Autodesk Fusion 360 part; units mm, degrees
sketch "草图1" plane through (0, 0, 0) normal (1, 0, 0) x (0, 1, 0)
  circle A0 centre (0, 0) radius 5
  circle A1 centre (0, 0) radius 11
  line L0 (0, 11) -> (62.4602, 11)
  line L1 (62.4602, 11) -> (44, -11)
  line L2 (44, -11) -> (0, -11)
  line L3 (62.4602, 11) -> (67.0565, 7.1433)
  line L4 (67.0565, 7.1433) -> (48.5963, -14.8567)
  line L5 (48.5963, -14.8567) -> (44, -11)
  dimension "d1" = 22
  dimension "d2" = 10
  dimension "d3" = 44
  dimension "d4" = 130
  dimension "d5" = 6
extrude "拉伸1" add sketch "草图1" along normal blind 19 contours A1 makes body 1
extrude "拉伸2" add sketch "草图1" along normal blind 5 contours A1 L0 L1 L2 bodies 1
extrude "拉伸3" add sketch "草图1" along normal blind 18 contours L1 L3 L4 L5 bodies 1
fillet "圆角1" radius 3 2 edges at (18, 64.7583, 9.0716) (18, 46.2981, -12.9284) on bodies 1
chamfer "倒角1" distance 1 angle 45 1 edges at (19, -4.6616, 1.8081) on bodies 1
sketch "草图2" plane through (0, 31.2367, -26.2107) normal (0, -0.766, 0.6428) x (1, 0, 0)
  arc A0 (15, 19.8562) -> (18, 22.8562) centre (15, 22.8562) ccw
  line L0 (18, 22.8562) -> (18, 45.5751)
  arc A1 (18, 45.5751) -> (15, 48.5751) centre (15, 45.5751) ccw
  line L1 (15, 48.5751) -> (5, 48.5751)
  line L2 (5, 48.5751) -> (5, 19.8562)
  line L3 (5, 19.8562) -> (15, 19.8562)
  line L4 (18, 34.2156) -> (5, 34.2156) construction
  circle A2 centre (12, 40.7156) radius 3.5
  circle A3 centre (12, 40.7156) radius 2.5
  circle A4 centre (12, 27.7156) radius 3.5
  circle A5 centre (12, 27.7156) radius 2.5
  dimension "d15" = 7
  dimension "d16" = 5
  dimension "d17" = 6
  dimension "d18" = 13
extrude "拉伸4" cut sketch "草图2" against normal blind 2 contours A2 | A4 bodies 1
extrude "拉伸5" cut 2 faces at (13.1784, 57.6864, 5.3108) (12.6885, 49.3537, -4.6197) along direction (0, 0.766044, -0.642788) blind 50 on bodies 1 bodies 1
sketch "草图3" plane through (0, 0, 0) normal (0, 0, 1) x (1, 0, 0)
  line L0 (5, 27) -> (20.5885, 0)
  line L1 (20.5885, 0) -> (5, 0)
  line L2 (5, 0) -> (5, 27)
  dimension "d23" = 5
  dimension "d24" = 27
  dimension "d25" = 30
extrude "拉伸6" add sketch "草图3" along normal mid plane 4 separate body makes body 2
extrude "拉伸7" cut sketch "草图1" along normal blind 43 contours A0 bodies 2
combine "合并1" operation add target body 1 tool bodies 2
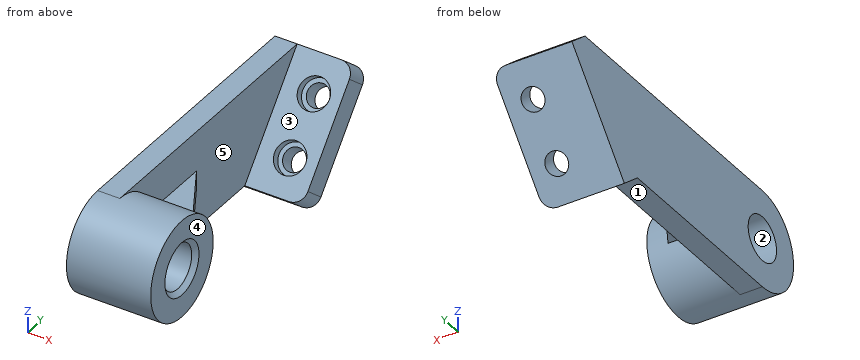
Work out the finished part from the listing and answer in its coordinate system (mm). Face numbers are marked on the shaded views. A direction names the side the tool comes from. Coordinates: 2 decimals unless noted, no trailing zeros. Loops run counter-clockwise (first coordinate to the right, second up) from the corner with the lowest first, then second, coordinate; pieces in that order, holes last. Notation, with made-up numbers: (61.25, -23.75) -> (113.25, -23.75) arc R20 cw to (113.25, -7.75) -> close; hole circle Ø5 at (69, 64.25). An arc over 180 degrees is marked (long way). Write each question's results on one line, items separated by ' | '. Start each with the question number.
1) Find section C-C on y = 30.5. Determine the outline of the cut face in (x, z).
2) For the marked faces 1, 2, 3, 4 and 5, determine the directions among +Z, -Z, +X, -X, +Y, -Y from which every point of the face is accessible in a straight line to the end or side of a thin tool.
3) Find section B-B on x = 11.75. Count the separate pieces of the cut face and the enclosed holes in it, then the cut area to 3 significant figures.
4) Flat-ended cylindrical pins translate along their axes: P1, Ø4, axis at x = 5.5, y = 17, coming from the -Z side; P2, Ø11, axis at y = 35.5, z = -4.5, coming from the +X side; P3, Ø3, axis at x = 7.5, y = 15, coming from the -Z side. Find the tip coordinate at first contact, or state that the pin passes through.
5) Consider line 1 along Z through (x, y) = (10.5, 0); line 2 along X through (y, z) = (19, -10.25); line 3 along Y through (x, z) = (13.25, 9). Determine where each line is inside the solid, lowest interval first.
6) Find section A-A on x = 7. Determine the outline of the cut face in (y, z), then the cut area to 3 significant figures.
Response values:
1) outline: (0, -11) -> (5, -11) -> (5, 11) -> (0, 11) -> close
2) face 1: -Z, +X, -X, -Y | face 2: +X, -X | face 3: +Z, +X | face 4: +Z, -Z, +X, +Y, -Y | face 5: +X
3) separate pieces: 4 | enclosed holes: 1 | area: 424 mm^2
4) P1: stops at z = -11 | P2: stops at x = 5 | P3: stops at z = -2
5) line 1: z = -11 to -5, 5 to 11 | line 2: x = 0 to 5 | line 3: y = -6.32 to 6.32, 60.78 to 64.84
6) outline: (10.82, -2) -> (23.54, -2) -> (23.54, 2) -> (10.82, 2) arc R11 ccw (long way) to start; (44, -11) -> (48.6, -14.86) -> (67.06, 7.14) -> (62.46, 11) -> close; hole circle Ø10 at (0, 0) | area: 524 mm^2
